Geometry check sheet. Reference: the model listing, model coordinates, mm. A direction names the side the tool comes from. Round coordinates to 2 decimals unless told otherwise and drop trailing zeros. Order: outer loops, then holes, each group sorted by start corner. A loop starts at its lowest first (then second) coordinate and runs counter-clockwise, first axis right, second up.
(1) Sectioned sample at B-B (z = 77). Record the boundary of the cut face in (x, y), plus the area to 3 significant figures.
(2) Go/stop test with flat-tipped pins: pin 1 (1.5 mm diameter, centred on x = 36, z = 47, fed in from -Y); pin 2 (1.5 mm diameter, centred on x = 19, y = 10, fed in from +Z); pin 3 (2 mm diameter, centred on y = 24, z = 52.5, fed in from -X). Record where each tip stops, or that it passes through.
(3) Sectioned sample at D-D (z = 24). Record the boundary of the cut face in (x, y), plus the area to 3 significant figures.
(4) Sectioned sample at C-C (x = 12.5). Record the boundary of the cut face in (y, z), plus the area to 3 significant figures.
(5) Release check for a two-part mould opening along Y. For faces 1 (the face through (62.58, -0.39, 9.86)), 2 (the face through (31, 23, 41)), 3 (the face through (47.591, 25.028, 27.395)), 4 (the face through (2.281, 20.594, 10.874)) record: +Y half, -Y half, draft (parallel to the pull), parting line (faces both ways), or undercut.
(6) Sectioned sample at A-A (y = 9.5). Record the boundary of the cut face in (x, z).
(7) Material ranges on line 1 along Y through (x, z) = (27.5, 4); line 2 along Y through (x, z) = (22, 63.5); line 3 along Z through (x, y) = (20, 18.5), recorded low to high.
(8) Set-up check for faces 5 (the face through (21, 25, 68)), 6 (the face through (59.594, 20.719, 10.874)), 7 (the face through (66, 12, 10)), 8 (the face through (41, 25, 67)): record each of +Z, -Z, +X, -X, +Y, -Y from which the full face is reachable in a straight line by a thin tool's end or side.
Autodesk Fusion 360 part; units mm, degrees
sketch "Schizzo1" plane through (0, 0, 0) normal (0, 0, 1) x (1, 0, 0)
  line L0 (0, 0) -> (62, 0) construction
  line L1 (62, 0) -> (62, 23) construction
  line L2 (62, 23) -> (0, 23) construction
  line L3 (0, 23) -> (0, 0) construction
  line L4 (31, 23) -> (31, 0) construction
  line L5 (62, 23) -> (54, 23) construction
  line L6 (54, 23) -> (54, 0) construction
  line L7 (0, 23) -> (8, 23) construction
  line L8 (8, 23) -> (8, 0) construction
  line L9 (8, 0) -> (54, 0)
  line L10 (8, 23) -> (54, 23)
  line L11 (0, 23) -> (0, 15) construction
  line L12 (0, 15) -> (62, 15) construction
  line L13 (0, 0) -> (0, 8) construction
  line L14 (0, 8) -> (62, 8) construction
  line L15 (0, 15) -> (0, 8) construction
  line L16 (0, 15) -> (0, 8)
  line L17 (62, 15) -> (62, 8)
  arc A0 (8, 23) -> (0, 15) centre (8, 15) ccw
  arc A1 (0, 8) -> (8, 0) centre (8, 8) ccw
  arc A2 (54, 0) -> (62, 8) centre (54, 8) ccw
  arc A3 (62, 15) -> (54, 23) centre (54, 15) ccw
  arc A4 (66, 15) -> (54, 27) centre (54, 15) ccw
  line L18 (8, 27) -> (54, 27)
  arc A5 (8, 27) -> (-4, 15) centre (8, 15) ccw
  line L19 (-4, 15) -> (-4, 8)
  arc A6 (-4, 8) -> (8, -4) centre (8, 8) ccw
  line L20 (8, -4) -> (54, -4)
  arc A7 (54, -4) -> (66, 8) centre (54, 8) ccw
  line L21 (66, 15) -> (66, 8)
  line L22 (0, 11.5) -> (62, 11.5) construction
  line L23 (0, 11.5) -> (-4, 11.5) construction
  line L24 (62, 11.5) -> (66, 11.5) construction
  dimension "d10" = 62
  dimension "d11" = 23
  dimension "d12" = 8
  dimension "d13" = 8
  dimension "d15" = 8
  dimension "d16" = 8
  dimension "d17" = -4
  dimension "d32" = 70
  dimension "d33" = 31
extrude "Estrusione2" add sketch "Schizzo1" along normal blind 20
extrude "Estrusione4" add sketch "Schizzo1" along normal blind 2 contours L9 L10 L16 L17 A0 A1 A2 A3
sketch "Schizzo3" plane through (0, 27, 0) normal (0, 1, 0) x (-1, 0, 0)
  line L0 (-54, 0) -> (-8, 0)
  line L1 (-8, 0) -> (-8, 20)
  line L2 (-8, 20) -> (-54, 20)
  line L3 (-54, 20) -> (-54, 0)
  line L4 (-31, 20) -> (-31, 100) construction
  line L5 (-31, 60) -> (-21, 60) construction
  line L6 (-21, 20) -> (-41, 20)
  line L7 (-41, 20) -> (-41, 100)
  line L8 (-41, 100) -> (-21, 100)
  line L9 (-21, 100) -> (-21, 20)
  line L10 (-21, 20) -> (-41, 100) construction
  line L11 (-41, 20) -> (-21, 100) construction
  point P0 (-31, 60)
  dimension "d22" = 20
  dimension "d23" = 80
extrude "Estrusione3" add sketch "Schizzo3" against normal blind 4 contours L2 L6 L7 L8 L9
sketch "Schizzo4" plane through (0, 27, 0) normal (0, 1, 0) x (-1, 0, 0)
  line L0 (-54, 0) -> (-8, 0)
  line L1 (-8, 0) -> (-8, 20)
  line L2 (-8, 20) -> (-21, 20)
  line L3 (-21, 20) -> (-21, 100)
  line L4 (-21, 100) -> (-41, 100)
  line L5 (-41, 100) -> (-41, 20)
  line L6 (-41, 20) -> (-54, 20)
  line L7 (-54, 20) -> (-54, 0)
  line L8 (-54, 20) -> (-41, 35)
  line L9 (-31, 100) -> (-31, -12.8301) construction
  line L10 (-8, 20) -> (-21, 35)
extrude "Estrusione5" add sketch "Schizzo4" against normal blind 4 contours L5 L6 L8 | L2 L3 L10
equation "d12 = d13"
equation "d15 = d13"
equation "d16 = d13"
Answer below:
1. outline: (21, 23) - (41, 23) - (41, 27) - (21, 27) - close
1. area: 80.0 mm2
2. pin 1: stops at y = 23
2. pin 2: stops at z = 2
2. pin 3: stops at x = 21
3. outline: (11.47, 23) - (50.53, 23) - (50.53, 27) - (11.47, 27) - close
3. area: 156 mm2
4. outline: (-4, 0) - (27, 0) - (27, 25.19) - (23, 25.19) - (23, 2) - (0, 2) - (0, 20) - (-4, 20) - close
4. area: 227 mm2
5. face 1: -Y half
5. face 2: undercut
5. face 3: draft
5. face 4: undercut
6. outline: (-4, 0) - (66, 0) - (66, 20) - (62, 20) - (62, 2) - (0, 2) - (0, 20) - (-4, 20) - close
7. line 1: y = -4 to 0, 23 to 27
7. line 2: y = 23 to 27
7. line 3: z = 0 to 2
8. face 5: +Z, -X, +Y, -Y
8. face 6: +Z
8. face 7: +Z, -Z, +X, +Y, -Y
8. face 8: +Z, +X, +Y, -Y
